from build123d import *

# Parameters (mm, degrees)
F1_DEPTH = 25


with BuildPart() as f1:
    # F0 (on Front) → F1 (new body)
    with BuildSketch(Plane.XZ):
        with BuildLine():
            Line((4, 30), (0, 0))
            Line((0, 0), (16, 0))
            Line((16, 0), (12, 30))
            ThreePointArc((12, 30), (13.101797, 33.321964), (16.39556, 34.505405))
            Line((16.39556, 34.505405), (58, 30))
            Line((58, 30), (46.895875, 43.801154))
            ThreePointArc((46.895875, 43.801154), (45.224745, 50.050887), (48.722404, 55.493149))
            Line((48.722404, 55.493149), (78, 74.814698))
            ThreePointArc((78, 74.814698), (73.172757, 79.252073), (72.131917, 85.725807))
            Line((72.131917, 85.725807), (75.002716, 102))
            Line((75.002716, 102), (58.728522, 99.129201))
            ThreePointArc((58.728522, 99.129201), (47.385802, 106.196158), (53.198466, 118.229948))
            Line((53.198466, 118.229948), (16.39556, 103.143887))
            Line((16.39556, 103.143887), (32.905704, 164.760587))
            ThreePointArc((32.905704, 164.760587), (23.68264, 157.358295), (13.84952, 163.928576))
            Line((13.84952, 163.928576), (8, 180))
            Line((8, 180), (2.15048, 163.928576))
            ThreePointArc((2.15048, 163.928576), (-7.68264, 157.358295), (-16.905704, 164.760587))
            Line((-16.905704, 164.760587), (-0.39556, 103.143887))
            Line((-0.39556, 103.143887), (-37.198466, 118.229948))
            ThreePointArc((-37.198466, 118.229948), (-31.385802, 106.196158), (-42.728522, 99.129201))
            Line((-42.728522, 99.129201), (-59.002716, 102))
            Line((-59.002716, 102), (-56.131917, 85.725807))
            ThreePointArc((-56.131917, 85.725807), (-57.172757, 79.252073), (-62, 74.814698))
            Line((-62, 74.814698), (-32.722404, 55.493149))
            ThreePointArc((-32.722404, 55.493149), (-29.224745, 50.050887), (-30.895875, 43.801154))
            Line((-30.895875, 43.801154), (-42, 30))
            Line((-42, 30), (-0.39556, 34.505405))
            ThreePointArc((-0.39556, 34.505405), (2.898203, 33.321964), (4, 30))
        make_face()
    extrude(amount=F1_DEPTH)


solid = f1.part
The listing builds one solid part. Answer for the finished solid, in the listing's coordinates (mm). A direction names the side the tool comes from. Give positions to 0.01 mm unless a question says otherwise; leave off trailing zeros. Order: outer loops, then holes, each group sorted by start corner. A loop starts at its lowest first (then second) coordinate and runs counter-clockwise, first axis right, second up. Notation, with made-up numbers: (45, 27) - (66, 27) arc R26 ccw to (66, 64) - close; hole circle Ø11 at (50, 40.5). An arc over 180 degrees is marked (long way). One line per item, written item: value. Start each with the question number.
1) A cutting plane is placed at C-C on z = 13.5. Give the vertices of the cut face in (x, y), then the cut area to 3 significant figures.
2) The mould has two halves that part along X. Classify faces 1 (the face through (36.907, -12.325, 32.284)), 2 (the face through (52.53, -12.32, 36.8)), 3 (the face through (7, 0, 91)): released by +X, released by -X, zero draft, split by the parting line, or undercut.
3) A tool of negligible diameter and unlimited length cuts with its end or side. For faces 4 (the face through (73.547, -12.325, 93.749)), 5 (the face through (-47.57, -12.32, 65.29)), 6 (the face through (66.98, -12.325, 100.585)), 7 (the face through (24.535, -12.325, 133.521)), 8 (the face through (-21.49, -12.32, 32.22)), from which of +Z, -Z, +X, -X, +Y, -Y can it reach the whole face along a straight path? Write none if from no direction.
4) Given pin 1 Ø12 at (x, z) = (38.5, 109.5) entering from +Y; pin 2 Ø4 at (x, y) = (-27.5, -13.5) entering from -Z; pin 3 Ø3 at (x, y) = (22, -8.5) entering from -Z; pin 4 Ø1.5 at (y, z) = (-14.5, 159) entering from +X, each flat-ended and moving along its own axis, determine where each tip first touches the part or whether it passes through.
5) Find the intervals of material crossed by L1, parallel to Z at x = -32.5, y = -6.75; L2, parallel to Z at x = -34, y = -21.5; L3, parallel to Z at x = -40, y = -4.5, in increasing order.
6) A cutting plane is placed at D-D on x = -39.5. Give the vertices of the cut face in (y, z), then the cut area to 3 significant figures.
7) A cutting plane is placed at A-A on x = 29.5. Give the vertices of the cut face in (y, z), then the cut area to 3 significant figures.
Answer sheet:
1. outline: (1.8, -25) - (14.2, -25) - (14.2, 0) - (1.8, 0) - close
1. area: 310 mm2
2. face 1: undercut
2. face 2: released by +X
2. face 3: zero draft
3. face 4: +X, +Y, -Y
3. face 5: -X, +Y, -Y
3. face 6: +Z, +Y, -Y
3. face 7: +Y, -Y
3. face 8: -Z, +Y, -Y
4. pin 1: stops at y = 0
4. pin 2: stops at z = 31.35
4. pin 3: stops at z = 33.74
4. pin 4: stops at x = 31.56
5. L1: z = 31.03 to 41.81, 55.34 to 103.7, 114.26 to 116.3
5. L2: z = 30.87 to 39.94, 56.34 to 101.83, 116.13 to 116.92
5. L3: z = 30.22 to 32.49, 60.3 to 99.03
6. outline: (-25, 30.27) - (0, 30.27) - (0, 33.11) - (-25, 33.11) - close; (-25, 59.97) - (0, 59.97) - (0, 99.09) - (-25, 99.09) - close
6. area: 1,050 mm2
7. outline: (-25, 33.09) - (0, 33.09) - (0, 108.52) - (-25, 108.52) - close; (-25, 152.05) - (0, 152.05) - (0, 159.55) - (-25, 159.55) - close
7. area: 2,070 mm2
